Can you work these out from the model? Positions are in its coordinate system, mm. A direction names the side the tool comes from. Coordinates: 2 decimals unless noted, no trailing zeros. Loops run counter-clockwise (first coordinate to the right, second up) from the corner with the lowest first, then second, coordinate; pieces in that order, holes last. Notation, with made-up numbers: M 12.5,75 L 51.5,75 A18 ccw 51.5,103 Z; hole C 57,13.5 d6. An arc over 180 degrees is marked long. Answer as a JSON object with one key per item and string values. Group by question number.
Item 1: Which directions (+Z, -Z, +X, -X, +Y, -Y) give clear straight access to the entire face, cutting with the end or side of a thin tool? Please do faces 4 (the cylindrical face through (-31.75, -16.08, -11.58)), 5 (the flat face through (17, -20, 0)).
Item 2: Suppose I cut it at C-C (y = -44). Write out the boundary of the cut face in (x, z).
Item 3: If I drill on line 1 (Y direction, x = 0, z = -2.7); line 2 (X direction, y = 0, z = -15.5); line 3 (X direction, y = -16.5, z = -1.7), over which ranges is the centre line in solid material (lowest first)?
Item 4: Suppose I cut it at B-B (y = 33). Write out the boundary of the cut face in (x, z).
Item 5: We'd pull the mould along Y, two halves only. Please class faces 1 (the flat face through (0, 0, 1)), 2 (the flat face through (-16.4, -9.7, 0)), 3 (the flat face through (8, -60, -8)): +Y half, -Y half, draft (parallel to the pull), parting line (faces both ways), or undercut.
Item 6: Suppose I cut it at A-A (y = -18). Write out the boundary of the cut face in (x, z).
Item 7: I'm going to push flat-ended pins straight in: pin 1 Ø14.5 at (x, y) = (0, 33) entering from +Z; pin 2 Ø4.5 at (x, y) = (11.26, -6.5) entering from +Z; pin 3 Ø3 at (y, z) = (7.5, -14.5) entering from +X. Where does each tip first touch, or does it pass through?
Autodesk Inventor part; units mm, degrees
ref_plane "YZ Plane" through (0, 0, 0) normal (1, 0, 0) x (0, 1, 0)
ref_plane "XZ Plane" through (0, 0, 0) normal (0, 1, 0) x (-1, 0, 0)
ref_plane "XY Plane" through (0, 0, 0) normal (0, 0, 1) x (1, 0, 0)
sketch "スケッチ1" plane through (0, 0, 0) normal (0, 0, 1) x (1, 0, 0)
  arc A0 (40, 0) -> (-24, -32) centre (0, 0) ccw
  line L0 (40, 0) -> (-24, 0)
  line L1 (-24, -32) -> (-24, -60)
  line L2 (-24, -60) -> (40, -60)
  line L3 (40, -60) -> (40, 0)
  circle A1 centre (0, 0) radius 33
  line L4 (-22, 0) -> (-11, 19.0526)
  line L5 (-11, 19.0526) -> (11, 19.0526)
  line L6 (11, 19.0526) -> (22, 0)
  line L7 (22, 0) -> (11, -19.0526)
  line L8 (11, -19.0526) -> (-11, -19.0526)
  line L9 (-11, -19.0526) -> (-22, 0)
  line L10 (-13, -25.5275) -> (13, -25.5275)
  line L11 (13, -25.5275) -> (29.4764, 3.0105)
  line L12 (29.4764, 3.0105) -> (16.4764, 25.5271)
  line L13 (16.4764, 25.5271) -> (-16.4764, 25.5271)
  line L14 (-16.4764, 25.5271) -> (-29.4764, 3.0105)
  line L15 (-29.4764, 3.0105) -> (-13, -25.5275)
  point P0 (-24, -32)
  point P1 (0, 33)
  point P2 (-28.5788, -16.5)
  point P3 (28.5788, -16.5)
  dimension "d34" = 66
  dimension "d0" = 80
  dimension "d1" = 0
  dimension "d2" = 64
  dimension "d3" = 60
  dimension "d35" = 0
  dimension "d38" = 360
  dimension "d62" = 22
  dimension "d94" = 0
  dimension "d95" = 26
  dimension "d96" = 120
  dimension "d97" = 26
  dimension "d98" = 120
  dimension "d99" = 120
  dimension "d100" = 26
  dimension "d101" = 120
  dimension "d102" = 13
  dimension "d103" = 25.5275
extrude "押し出し1" add sketch "スケッチ1" against normal blind 17 contours L3 L2 L1 A0 | L7 L8 L9 L0 | L0 L4 L5 L6 | L11 L10 L15 L14 L13 L12 | A1
hole "穴3" at (0, 33, 0) at (-28.5788, -16.5, 0) at (28.5788, -16.5, 0) direction (0, 0, -1) diameter 6.4 depth 17 tip angle 118 counterbore diameter 11 counterbore depth 6
sketch "スケッチ2" plane through (0, 0, -17) normal (0, 0, -1) x (-1, 0, 0)
  circle A0 centre (0, 0) radius 35
  point P0 (-35, 0)
  point P1 (35, 0)
  dimension "d47" = 70
  dimension "d48" = 0
  dimension "d51" = 360
hole "穴4" at (35, 0, -17) at (-35, 0, -17) direction (0, 0, 1) diameter 4 depth 4 tip angle 118
extrude "押し出し2" add sketch "スケッチ1" along normal blind 1 contours L7 L8 L9 L0 | L0 L4 L5 L6
sketch "スケッチ4" plane through (0, 0, 1) normal (0, 0, 1) x (1, 0, 0)
  circle A0 centre (0, 0) radius 13
  point P0 (0, 13)
  point P1 (-11.2583, -6.5)
  point P2 (11.2583, -6.5)
  dimension "d81" = 26
  dimension "d82" = 0
  dimension "d85" = 360
hole "穴5" at (0, 13, 1) at (-11.2583, -6.5, 1) at (11.2583, -6.5, 1) direction (0, 0, -1) diameter 4.917 depth 10 tip angle 118
extrude "押し出し3" cut sketch "スケッチ1" against normal blind 1 contours L11 L10 L15 L14 L13 L12
properties part number "FFS080YS102U6" material "ステンレス鋼"
From the geometry:
{
 "1": {"face 4": "+Z, -Z", "face 5": "+Z"},
 "2": {"outline": "M -24,-17 L 40,-17 L 40,0 L -24,0 Z"},
 "3": {"line 1": "-60 to 10.54, 15.46 to 27.5, 38.5 to 40", "line 2": "-40 to -37, -33 to 33, 37 to 40", "line 3": "-36.44 to -34.08, -23.08 to 23.08, 34.08 to 40"},
 "4": {"outline": "M -22.61,-17 L -3.2,-17 L -3.2,-6 L -5.5,-6 L -5.5,0 L -22.61,0 Z; M 3.2,-17 L 22.61,-17 L 22.61,0 L 5.5,0 L 5.5,-6 L 3.2,-6 Z"},
 "5": {"face 1": "draft", "face 2": "undercut", "face 3": "-Y half"},
 "6": {"outline": "M -35.72,-17 L -31.41,-17 L -31.41,-6 L -33.87,-6 L -33.87,0 L -35.72,0 Z; M -25.75,-17 L 25.75,-17 L 25.75,-6 L 23.29,-6 L 23.29,0 L 17.35,0 L 17.35,-1 L 11.61,-1 L 11.61,1 L -11.61,1 L -11.61,-1 L -17.35,-1 L -17.35,0 L -23.29,0 L -23.29,-6 L -25.75,-6 Z; M 31.41,-17 L 40,-17 L 40,0 L 33.87,0 L 33.87,-6 L 31.41,-6 Z"},
 "7": {"pin 1": "z = 0", "pin 2": "z = -9.12", "pin 3": "x = 39.55"}
}
